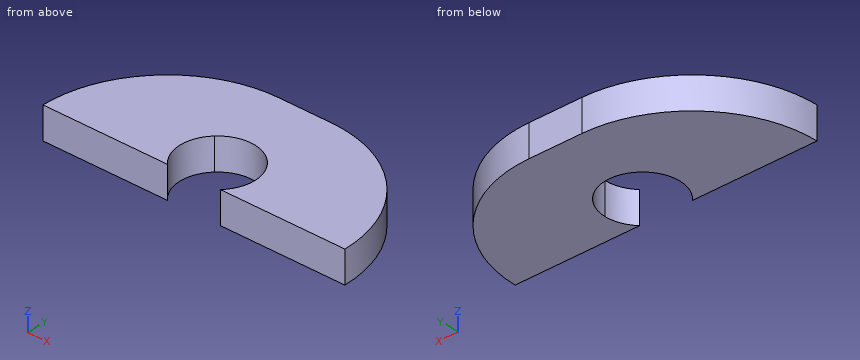
from build123d import *

# Parameters (mm, degrees)
F1_DEPTH = 5


with BuildPart() as f1:
    # F0 (on Top) → F1 (new body)
    with BuildSketch(Plane.XY):
        with BuildLine():
            ThreePointArc((5.8520560333, -5.611971495), (5.4065947922, -7.8514563842), (4.138028505, -9.75))
            Line((4.138028505, -9.75), (9.8424661541, -9.75))
            Line((9.8424661541, -9.75), (12.414085515, -9.75))
            ThreePointArc((12.414085515, -9.75), (9.9900845383, -3.8979439667), (4.138028505, -1.47394299))
            ThreePointArc((4.138028505, -1.47394299), (5.4065947922, -3.3724866058), (5.8520560333, -5.611971495))
        make_face()
        with BuildLine():
            Line((-12.414085515, -9.75), (-4.138028505, -9.75))
            ThreePointArc((-4.138028505, -9.75), (-5.8520560333, -5.611971495), (-4.138028505, -1.47394299))
            ThreePointArc((-4.138028505, -1.47394299), (-9.9900845383, -3.8979439667), (-12.414085515, -9.75))
        make_face()
        with BuildLine():
            ThreePointArc((-4.138028505, -1.47394299), (0, 0.2400845383), (4.138028505, -1.47394299))
            Line((4.138028505, -1.47394299), (4.138028505, 7.9066384221))
            ThreePointArc((4.138028505, 7.9066384221), (2.1083185822, 8.7224970718), (0, 9.305884133))
            ThreePointArc((0, 9.305884133), (-2.1083185822, 8.7224970718), (-4.138028505, 7.9066384221))
            Line((-4.138028505, 7.9066384221), (-4.138028505, -1.47394299))
        make_face()
        with BuildLine():
            Line((4.138028505, 7.9066384221), (4.138028505, -1.47394299))
            ThreePointArc((4.138028505, -1.47394299), (9.9900845383, -3.8979439667), (12.414085515, -9.75))
            Line((12.414085515, -9.75), (15.361971495, -9.75))
            ThreePointArc((15.361971495, -9.75), (12.3184764656, 0.7110441234), (4.138028505, 7.9066384221))
        make_face()
        with BuildLine():
            ThreePointArc((-12.414085515, -9.75), (-9.9900845383, -3.8979439667), (-4.138028505, -1.47394299))
            Line((-4.138028505, -1.47394299), (-4.138028505, 7.9066384221))
            ThreePointArc((-4.138028505, 7.9066384221), (-12.3184764656, 0.7110441234), (-15.361971495, -9.75))
            Line((-15.361971495, -9.75), (-12.414085515, -9.75))
        make_face()
        with BuildLine():
            ThreePointArc((0, 9.305884133), (2.1083185822, 8.7224970718), (4.138028505, 7.9066384221))
            Line((4.138028505, 7.9066384221), (4.138028505, 9.75))
            ThreePointArc((4.138028505, 9.75), (2.057132135, 9.6386531326), (0, 9.305884133))
        make_face()
        with BuildLine():
            Line((4.138028505, 9.75), (4.138028505, 7.9066384221))
            ThreePointArc((4.138028505, 7.9066384221), (12.3184764656, 0.7110441234), (15.361971495, -9.75))
            Line((15.361971495, -9.75), (23.638028505, -9.75))
            ThreePointArc((23.638028505, -9.75), (17.9266107381, 4.0385822331), (4.138028505, 9.75))
        make_face()
        with BuildLine():
            ThreePointArc((-15.361971495, -9.75), (-12.3184764656, 0.7110441234), (-4.138028505, 7.9066384221))
            Line((-4.138028505, 7.9066384221), (-4.138028505, 9.75))
            ThreePointArc((-4.138028505, 9.75), (-17.9266107381, 4.0385822331), (-23.638028505, -9.75))
            Line((-23.638028505, -9.75), (-15.361971495, -9.75))
        make_face()
        with BuildLine():
            Line((-4.138028505, 9.75), (-4.138028505, 7.9066384221))
            ThreePointArc((-4.138028505, 7.9066384221), (-2.1083185822, 8.7224970718), (0, 9.305884133))
            ThreePointArc((0, 9.305884133), (-2.057132135, 9.6386531326), (-4.138028505, 9.75))
        make_face()
        with BuildLine():
            ThreePointArc((0, 9.305884133), (2.057132135, 9.6386531326), (4.138028505, 9.75))
            Line((4.138028505, 9.75), (-4.138028505, 9.75))
            ThreePointArc((-4.138028505, 9.75), (-2.057132135, 9.6386531326), (0, 9.305884133))
        make_face()
    extrude(amount=F1_DEPTH)


solid = f1.part
Read the model definition and answer for the solid it produces. Units are mm, in the model's axes. Coordinates: 2 decimals unless noted, no trailing zeros. Loops run counter-clockwise (first coordinate to the right, second up) from the corner with the lowest first, then second, coordinate; pieces in that order, holes last. Notation, with made-up numbers: (81.5, 89.5) -> (125.5, 89.5) arc R30 ccw to (125.5, 120.5) -> close; hole circle Ø4 at (66, 55). An arc over 180 degrees is marked (long way). Write item = value, one per line. Start each with the question number.
1) The part is cut by section D-D, the plane x = -13. Determine the outline of the cut face in (y, z).
2) Given P1, Ø2, axis at y = 5, z = 2, coming from the -X side; P2, Ø2, axis at x = -13.5, z = 3, coming from the +Y side, each flat-ended and moving along its own axis, determine where each tip first touches the part or whether it passes through.
3) The part is cut by section B-B, the plane z = 3.85. Determine the outline of the cut face in (x, y), plus the area to 3 significant figures.
4) The part is cut by section C-C, the plane y = -8. Determine the outline of the cut face in (x, z), plus the area to 3 significant figures.
5) Find the intervals of material crossed by L1, parallel to Y at x = 0, z = 3.6; L2, parallel to X at y = -2.75, z = 2.05; L3, parallel to X at y = -7.5, z = 1.2, in increasing order. Write a range as from..to.
6) The part is cut by section A-A, the plane y = -4.5. Determine the outline of the cut face in (x, z), plus the area to 3 significant figures.
Result:
q1.outline = (-9.75, 0) -> (7.62, 0) -> (7.62, 5) -> (-9.75, 5) -> close
q2.P1 = -17.97
q2.P2 = 7.87
q3.outline = (-23.64, -9.75) -> (-4.14, -9.75) arc R5.85 cw (long way) to (4.14, -9.75) -> (23.64, -9.75) arc R19.5 ccw to (4.14, 9.75) -> (-4.14, 9.75) arc R19.5 ccw to start
q3.area = 661 mm²
q4.outline = (-23.56, 0) -> (-5.34, 0) -> (-5.34, 5) -> (-23.56, 5) -> close; (5.34, 0) -> (23.56, 0) -> (23.56, 5) -> (5.34, 5) -> close
q4.area = 182 mm²
q5.L1 = 0.24..9.75
q5.L2 = -22.34..-5.1, 5.1..22.34
q5.L3 = -23.51..-5.54, 5.54..23.51
q6.outline = (-22.92, 0) -> (-5.75, 0) -> (-5.75, 5) -> (-22.92, 5) -> close; (5.75, 0) -> (22.92, 0) -> (22.92, 5) -> (5.75, 5) -> close
q6.area = 172 mm²
